Here's how the part is built. I have some questions about the finished solid (model axes, mm). Face numbers are marked on the shaded views. A direction names the side the tool comes from. Round coordinates to 2 decimals unless told otherwise and drop trailing zeros. Order: outer loops, then holes, each group sorted by start corner. A loop starts at its lowest first (then second) coordinate and runs counter-clockwise, first axis right, second up. Notation, with made-up numbers: M 64.5,64 L 106.5,64 A18 ccw 106.5,98 Z; hole C 26,-12.5 d11. An arc over 180 degrees is marked long. Answer as CSV lines item,"result". Start each with the question number.
Autodesk Inventor part; units mm, degrees
ref_plane "YZ Plane" through (0, 0, 0) normal (1, 0, 0) x (0, 1, 0)
ref_plane "XZ Plane" through (0, 0, 0) normal (0, 1, 0) x (-1, 0, 0)
ref_plane "XY Plane" through (0, 0, 0) normal (0, 0, 1) x (1, 0, 0)
sketch "草图1" plane through (0, 0, 0) normal (0, 0, 1) x (1, 0, 0)
  circle A0 centre (0, 0) radius 27.5
  line L0 (27.5, 0) -> (19.8431, 2.5)
  line L1 (0, 0) -> (42.7409, 0) construction
  line L2 (27.5, 0) -> (19.8431, -2.5)
  line L3 (19.4454, 19.4454) -> (12.2634, 15.799)
  line L4 (19.4454, 19.4454) -> (15.799, 12.2634)
  line L5 (0, 27.5) -> (-2.5, 19.8431)
  line L6 (0, 27.5) -> (2.5, 19.8431)
  line L7 (-19.4454, 19.4454) -> (-15.799, 12.2634)
  line L8 (-19.4454, 19.4454) -> (-12.2634, 15.799)
  line L9 (-27.5, 0) -> (-19.8431, -2.5)
  line L10 (-27.5, 0) -> (-19.8431, 2.5)
  line L11 (-19.4454, -19.4454) -> (-12.2634, -15.799)
  line L12 (-19.4454, -19.4454) -> (-15.799, -12.2634)
  line L13 (0, -27.5) -> (2.5, -19.8431)
  line L14 (0, -27.5) -> (-2.5, -19.8431)
  line L15 (19.4454, -19.4454) -> (15.799, -12.2634)
  line L16 (19.4454, -19.4454) -> (12.2634, -15.799)
  arc A1 (19.8431, 2.5) -> (15.799, 12.2634) centre (0, 0) ccw
  arc A2 (15.799, -12.2634) -> (19.8431, -2.5) centre (0, 0) ccw
  arc A3 (2.5, -19.8431) -> (12.2634, -15.799) centre (0, 0) ccw
  arc A4 (-12.2634, -15.799) -> (-2.5, -19.8431) centre (0, 0) ccw
  arc A5 (-19.8431, -2.5) -> (-15.799, -12.2634) centre (0, 0) ccw
  arc A6 (-15.799, 12.2634) -> (-19.8431, 2.5) centre (0, 0) ccw
  arc A7 (12.2634, 15.799) -> (2.5, 19.8431) centre (0, 0) ccw
  arc A8 (-2.5, 19.8431) -> (-12.2634, 15.799) centre (0, 0) ccw
  dimension "d1" = 55
  dimension "d2" = 2.5
  dimension "d5" = 360
extrude "拉伸1" add sketch "草图1" along normal blind 62 contours L2 A2 L15 L16 A3 L13 L14 A4 L11 L12 A5 L9 L10 A6 L7 L8 A8 L5 L6 A7 L3 L4 A1 L0
sketch "草图2" plane through (0, 0, 62) normal (0, 0, 1) x (1, 0, 0)
  circle A0 centre (0, 0) radius 15
  dimension "d9" = 30
extrude "拉伸2" cut sketch "草图2" against normal through all
fillet "圆角1" radius 0.3 8 edges at (19.4454, 19.4454, 31) (0, 27.5, 31) (27.5, 0, 31) (19.4454, -19.4454, 31) (0, -27.5, 31) (-15.8544, -17.6222, 62) (-27.5, 0, 31) (-19.4454, 19.4454, 31)
properties part number "滚轮设计" material "橡胶"
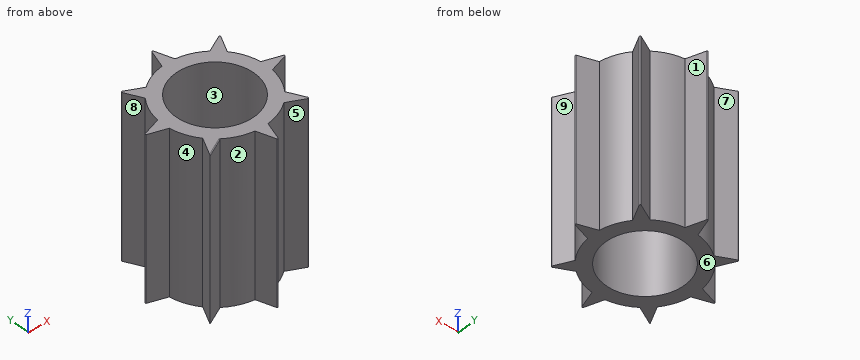
Item 1: For P1, Ø1, axis at x = 15, z = 47, coming from the +Y side; P2, Ø12, axis at y = -21, z = 7, coming from the +X side; P3, Ø8, axis at x = -18, z = 28.5, coming from the +Y side, each with a flat end and sliding along its axis, tell me the tip position at first contact or that it passes through.
Item 2: If we section it at C-C on y = 13.5: Please give me the cut outline in (x, z).
Item 3: If we section it at A-A on y = 8: Please give me the cut outline in (x, z), and give its area (3 significant figures).
Item 4: If we section it at D-D on x = 22: Please give me the cut outline in (y, z), and give its area (3 significant figures).
Item 5: We'd pull the mould along X, two halves only. Please class the marked faces 1, 2, 3 and 4: pulls with the +X half, pulls with the -X half, needs draft (parallel to the pull), parting line crosses it, or undercut.
Item 6: If I drill on line 1 along Y through (x, z) = (-17, 8); line 2 along X through (y, z) = (6.5, 24.5); line 3 along X through (y, z) = (-16, 16), over which ranges is the centre line in solid material (lowest first)?
Item 7: Which directions (+Z, -Z, +X, -X, +Y, -Y) give clear straight access to the entire face, cutting with the end or side of a thin tool? Please do the marked faces 5, 6, 7, 8 and 9.
Geometry says:
1,P1,"y = 17.44"
1,P2,"x = 19.06"
1,P3,"y = 19.06"
2,outline,"M -16.43,0 L -6.54,0 L -6.54,62 L -16.43,62 Z; M 6.54,0 L 16.43,0 L 16.43,62 L 6.54,62 Z"
3,outline,"M -18.33,0 L -12.69,0 L -12.69,62 L -18.33,62 Z; M 12.69,0 L 18.33,0 L 18.33,62 L 12.69,62 Z"
3,area,"700 mm²"
4,outline,"M -1.8,0 L 1.8,0 L 1.8,62 L -1.8,62 Z"
4,area,"223 mm²"
5,face 1,"pulls with the +X half"
5,face 2,"undercut"
5,face 3,"undercut"
5,face 4,"pulls with the -X half"
6,line 1,"-18.2 to -14.63, -10.54 to 10.54, 14.63 to 18.2"
6,line 2,"-18.91 to -13.52, 13.52 to 18.91"
6,line 3,"-17.7 to -12.66, -12 to 12, 12.66 to 17.7"
7,face 5,"+Z, -Z, -Y"
7,face 6,"-Z, +X, -X, +Y, -Y"
7,face 7,"+Z, -Z, +Y"
7,face 8,"+Z, -Z, -X"
7,face 9,"+Z, -Z, +X"
